Part model, mm, in its own coordinate system. Give positions to 0.01 mm unless a question says otherwise; leave off trailing zeros. Order: outer loops, then holes, each group sorted by start corner. A loop starts at its lowest first (then second) coordinate and runs counter-clockwise, first axis right, second up. Notation, with made-up numbers: M -26,68.5 L 25,68.5 A24 cw 25,95.5 Z; hole C 78.5,-20.5 d7. An arc over 180 degrees is marked long. Answer as a JSON object with one key per item and string values.
from build123d import *

# Parameters (mm, degrees)
SKETCH_1_W          = 80
SKETCH_1_H          = 20
EXTRUDE_1_DEPTH     = 2
SKETCH_2_R          = 5
CUT_EXTRUDE_1_DEPTH = 42.279534881
SKETCH_3_W          = 80
SKETCH_3_H          = 2
EXTRUDE_2_DEPTH     = 40


with BuildPart() as part:
    # Эскиз1 → Бобышка-Вытянуть1 (new body)
    with BuildSketch(Plane.XY):
        Rectangle(SKETCH_1_W, SKETCH_1_H)
    extrude(amount=EXTRUDE_1_DEPTH)

    # Эскиз2 → Вырез-Вытянуть1 (cut, through all)
    with BuildSketch(Plane.XY.offset(2)):
        Circle(SKETCH_2_R)
    extrude(amount=-CUT_EXTRUDE_1_DEPTH, mode=Mode.SUBTRACT)

    # Эскиз3 → Бобышка-Вытянуть2 (add)
    with BuildSketch(Plane.XZ.offset(10)):
        with Locations((0, 1)):
            Rectangle(SKETCH_3_W, SKETCH_3_H)
    extrude(amount=EXTRUDE_2_DEPTH)


solid = part.part
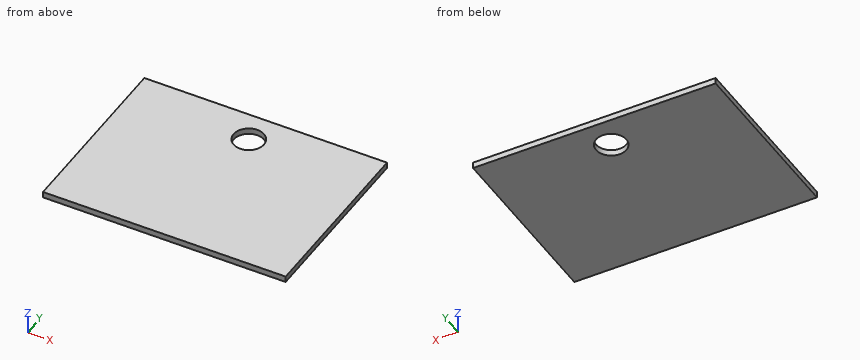
1. Cut at A-A on x = 0. Give the cut face in (y, z).
Worked answers:
{"outline": "M -50,0 L -5,0 L -5,2 L -50,2 Z; M 5,0 L 10,0 L 10,2 L 5,2 Z"}
2. Cut at C-C on z = 0.95. Give the cut face in (x, y), plus the area to 3 significant figures.
Worked answers:
{"outline": "M -40,-50 L 40,-50 L 40,10 L -40,10 Z; hole C 0,0 d10", "area": "4,720 mm^2"}
3. Probe line 1 along Y through (x, z) = (0, 1.55); line 2 along X through (y, z) = (3, 1.1); line 3 along X through (y, z) = (0.5, 1.3). List the from-to ranges inside material, lowest first.
Worked answers:
{"line 1": "y = -50 to -5, 5 to 10", "line 2": "x = -40 to -4, 4 to 40", "line 3": "x = -40 to -4.97, 4.97 to 40"}
4. Cut at B-B on y = 0. Give the cut face in (x, z).
Worked answers:
{"outline": "M -40,0 L -5,0 L -5,2 L -40,2 Z; M 5,0 L 40,0 L 40,2 L 5,2 Z"}
